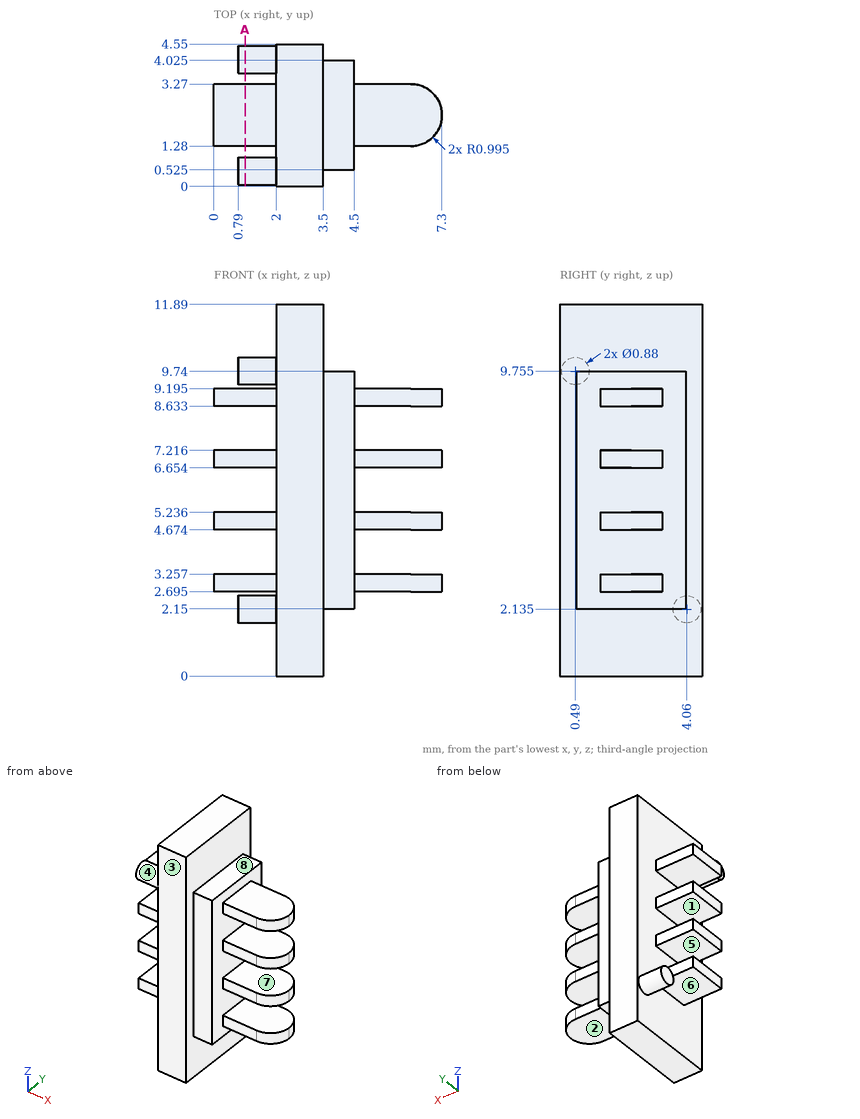
Geometry: see drawing. Coordinates: mm, zero at the bounding-box minimum. A direction names the side the tool comes from. Round coordinates to 2 decimals unless told otherwise and drop trailing zeros. Order: outer loops, then holes, each group sorted by start corner. A loop starts at its lowest first (then second) coordinate and runs counter-clockwise, first axis right, second up. Notation, with made-up numbers: (-10.5, 60) - (-4.5, 60) arc R19 cw to (-4.5, 73) - close; hole circle Ø8 at (53.25, 79.25). An arc over 180 degrees is marked (long way). Use a Markdown table: item, result. Add a question column.
1. First-contact query: pin 1 (0.6 mm diameter, centred on x = 5, z = 7, fed in from +Y); pin 2 (1.6 mm diameter, centred on x = 6, y = 2, fed in from -Z) (1 decimal); pin 3 (0.8 mm diameter, centred on x = 4, y = 2, fed in from +Z). Flat tips, straight axial feed; report the tip coordinate or a pass-through.
2. Mould query, pull axis Z, two halves, no side actions, for the marked faces 1, 2 and 3. Classes: +Z half, -Z half, draft (parallel to the pull), parting line (faces both ways), or undercut.
3. Line query: probe 1 along Z at (x, y) = (5.25, 1.45) (1 decimal); probe 2 along X at (y, z) = (4.2, 4); probe 3 along X at (y, z) = (2, 6). Output: solid intervals per line, ascending.
4. Section query A-A (x = 1). Return the cut outline in (y, z) (1 decimal).
5. Set-up query: the marked faces 4, 5, 6, 7 and 8. Return all of +Z, -Z, +X, -X, +Y, -Y with unobstructed straight access to the full face (end or side cutting, diameter ignored); none if empty.
Derived:
| question | item | result |
|---|---|---|
| 1 | pin 1 | y = 3.27 |
| 1 | pin 2 | z = 2.7 |
| 1 | pin 3 | z = 9.74 |
| 2 | face 1 | undercut |
| 2 | face 2 | -Z half |
| 2 | face 3 | draft |
| 3 | probe 1 | 2.7 to 3.3, 4.7 to 5.2, 6.7 to 7.2, 8.6 to 9.2 |
| 3 | probe 2 | 2 to 3.5 |
| 3 | probe 3 | 2 to 4.5 |
| 4 | outline | circle Ø0.9 at (0.5, 9.8); (1.3, 2.7) - (3.3, 2.7) - (3.3, 3.3) - (1.3, 3.3) - close; (1.3, 4.7) - (3.3, 4.7) - (3.3, 5.2) - (1.3, 5.2) - close; (1.3, 6.7) - (3.3, 6.7) - (3.3, 7.2) - (1.3, 7.2) - close; (1.3, 8.6) - (3.3, 8.6) - (3.3, 9.2) - (1.3, 9.2) - close; circle Ø0.9 at (4.1, 2.1) |
| 5 | face 4 | -X |
| 5 | face 5 | -X, +Y, -Y |
| 5 | face 6 | -Z, -X, +Y, -Y |
| 5 | face 7 | +X, +Y, -Y |
| 5 | face 8 | +Z, +X, +Y, -Y |
